from build123d import *

# Parameters (mm, degrees)
F0_W     = 130
F0_H     = 123
F0_W_2   = 125
F0_H_2   = 85
F1_DEPTH = 8
F2_R     = 2.8435
F2_R_2   = 2.524436
F3_DEPTH = 25
F4_W     = 60.26917
F4_H     = 116
F5_DEPTH = 25
F6_R     = 9.5
F6_R_2   = 2.8435
F6_R_3   = 2.524436
F7_DEPTH = 8


with BuildPart() as f1:
    # F0 (on Front) → F1 (new body)
    with BuildSketch(Plane.XZ):
        Rectangle(F0_W, F0_H)
        Rectangle(F0_W_2, F0_H_2, mode=Mode.SUBTRACT)
    extrude(amount=F1_DEPTH)

    # F2 (on face) → F3 (cut)
    with BuildSketch(Plane.XZ.offset(8)):
        with Locations((-50, 56.25)):
            Circle(F2_R)
        with Locations((50, 56.25)):
            Circle(F2_R)
        with Locations((-50, -56.25)):
            Circle(F2_R_2)
        with Locations((50, -56.25)):
            Circle(F2_R)
    extrude(amount=-F3_DEPTH, mode=Mode.SUBTRACT)

    # F4 (on face) → F5 (cut)
    with BuildSketch(Plane.XZ.offset(8)):
        Rectangle(F4_W, F4_H)
    extrude(amount=-F5_DEPTH, mode=Mode.SUBTRACT)

    # F6 (on face) → F7 (join, through all)
    with BuildSketch(Plane(origin=(0, 0, 0), x_dir=(-1, 0, 0), z_dir=(0, 1, 0))):
        with Locations((-50, 56.25)):
            Circle(F6_R)
        with Locations((-50, 56.25)):
            Circle(F6_R_2, mode=Mode.SUBTRACT)
        with Locations((50, 56.25)):
            Circle(F6_R)
        with Locations((50, 56.25)):
            Circle(F6_R_2, mode=Mode.SUBTRACT)
        with Locations((-50, -56.25)):
            Circle(F6_R)
        with Locations((-50, -56.25)):
            Circle(F6_R_2, mode=Mode.SUBTRACT)
        with Locations((50, -56.25)):
            Circle(F6_R)
        with Locations((50, -56.25)):
            Circle(F6_R_3, mode=Mode.SUBTRACT)
    extrude(amount=-F7_DEPTH)


solid = f1.part
The listing builds one solid part. Answer for the finished solid, in the listing's coordinates (mm). A direction names the side the tool comes from. Give positions to 0.01 mm unless a question says otherwise; leave off trailing zeros. Order: outer loops, then holes, each group sorted by start corner. A loop starts at its lowest first (then second) coordinate and runs counter-clockwise, first axis right, second up. Notation, with made-up numbers: (66.25, 13.5) -> (118.25, 13.5) arc R30 ccw to (118.25, 43.5) -> close; hole circle Ø1 at (47.25, -31.5). An arc over 180 degrees is marked (long way). Put each result on its own line as item: value.
Item 1: Given P1, Ø6.5, axis at x = 50, z = 56.25, coming from the +Y side; P2, Ø2.5, axis at x = 43.5, y = -6, coming from the -Z side; P3, Ø1.5, axis at x = 29.5, y = -3, coming from the +Z side; P4, Ø3.5, axis at x = 61.5, y = -3, coming from the -Z side, each flat-ended and moving along its own axis, determine where each tip first touches the part or whether it passes through.
Established:
P1: stops at y = 0
P2: stops at z = -64.17
P3: stops at z = 61.5
P4: stops at z = -61.5
Item 2: A cutting plane is placed at B-B on z = 56.25. Give the vertices of the cut face in (x, y), plus the area to 3 significant figures.
Established:
outline: (-65, -8) -> (-52.84, -8) -> (-52.84, 0) -> (-65, 0) -> close; (-47.16, -8) -> (-30.13, -8) -> (-30.13, 0) -> (-47.16, 0) -> close; (30.13, -8) -> (47.16, -8) -> (47.16, 0) -> (30.13, 0) -> close; (52.84, -8) -> (65, -8) -> (65, 0) -> (52.84, 0) -> close
area: 467 mm^2
Item 3: Straight lines are drawn through the part: line 1 (Z direction, x = -50, y = -2); line 2 (Z direction, x = 50, y = -4.5); line 3 (X direction, y = -4.5, z = -56.25). For each, find the intervals that lie inside material, in ascending order.
Established:
line 1: z = -65.75 to -58.77, -53.73 to -42.5, 42.5 to 53.41, 59.09 to 65.75
line 2: z = -65.75 to -59.09, -53.41 to -42.5, 42.5 to 53.41, 59.09 to 65.75
line 3: x = -65 to -52.52, -47.48 to -30.13, 30.13 to 47.16, 52.84 to 65
Item 4: For faces 4 (the face through (-1, -4, 61.5)), 5 (the face through (30.135, -4, -50)), 6 (the face through (-62, -4, -61.5)), determine the directions among +Z, -Z, +X, -X, +Y, -Y from which every point of the face is accessible in a straight line to the end or side of a thin tool.
Established:
face 4: +Z, +Y, -Y
face 5: +Y, -Y
face 6: -Z, -X, +Y, -Y
Item 5: A cutting plane is placed at C-C on y = -5.25. Give the vertices of the cut face in (x, z), plus the area to 3 significant figures.
Established:
outline: (-65, -61.5) -> (-57.92, -61.5) arc R9.5 ccw to (-42.08, -61.5) -> (42.08, -61.5) arc R9.5 ccw to (57.92, -61.5) -> (65, -61.5) -> (65, 61.5) -> (57.92, 61.5) arc R9.5 ccw to (42.08, 61.5) -> (-42.08, 61.5) arc R9.5 ccw to (-57.92, 61.5) -> (-65, 61.5) -> close; hole (-62.5, -42.5) -> (-30.13, -42.5) -> (-30.13, -58) -> (30.13, -58) -> (30.13, -42.5) -> (62.5, -42.5) -> (62.5, 42.5) -> (30.13, 42.5) -> (30.13, 58) -> (-30.13, 58) -> (-30.13, 42.5) -> (-62.5, 42.5) -> close; hole circle Ø5.69 at (-50, 56.25); hole circle Ø5.05 at (-50, -56.25); hole circle Ø5.69 at (50, -56.25); hole circle Ø5.69 at (50, 56.25)
area: 3,590 mm^2
Item 6: For a pull along Z with two mould halves and no side action, classify faces 1 (the face through (-62, -4, 61.5)), 2 (the face through (-47, -4, 42.5)), 3 (the face through (65, -4, -1)) as released by +Z, released by -Z, zero draft, split by the parting line, or undercut.
Established:
face 1: released by +Z
face 2: undercut
face 3: zero draft
Item 7: A cutting plane is placed at D-D on z = -51. Give the vertices of the cut face in (x, y).
Established:
outline: (-65, -8) -> (-30.13, -8) -> (-30.13, 0) -> (-65, 0) -> close; (30.13, -8) -> (65, -8) -> (65, 0) -> (30.13, 0) -> close
Item 8: A cutting plane is placed at A-A on x = 50. Give the vertices of the cut face in (y, z), plus the area to 3 significant figures.
Established:
outline: (-8, -65.75) -> (0, -65.75) -> (0, -59.09) -> (-8, -59.09) -> close; (-8, -53.41) -> (0, -53.41) -> (0, -42.5) -> (-8, -42.5) -> close; (-8, 42.5) -> (0, 42.5) -> (0, 53.41) -> (-8, 53.41) -> close; (-8, 59.09) -> (0, 59.09) -> (0, 65.75) -> (-8, 65.75) -> close
area: 281 mm^2
